from build123d import *

# Parameters (mm, degrees)
SKETCH_1_W      = 30
SKETCH_1_H      = 3
EXTRUDE_1_DEPTH = 3


with BuildPart() as part:
    # Эскиз1 → Бобышка-Вытянуть1 (new body)
    with BuildSketch(Plane.XY):
        Polygon((-25, 50), (-25, -50), (25, -50), (25, 50), (15, 50), (15, 47), (-15, 47), (-15, 50), align=None)
        with Locations((0, 48.5)):
            Rectangle(SKETCH_1_W, SKETCH_1_H)
        with Locations((0, 51.5)):
            Rectangle(SKETCH_1_W, SKETCH_1_H)
    extrude(amount=EXTRUDE_1_DEPTH)


solid = part.part
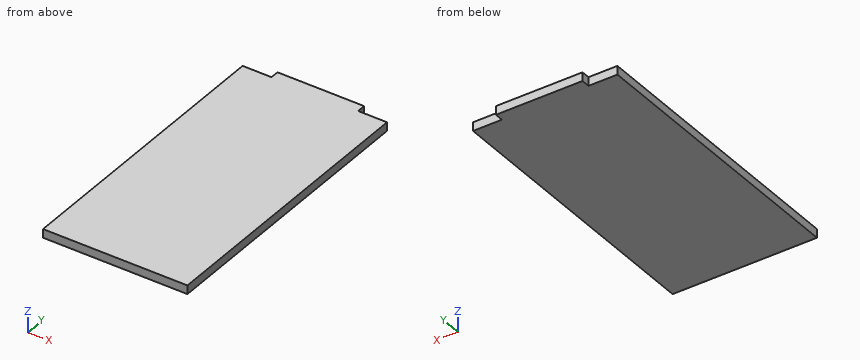
CAD build for the part. Positions are in the model's coordinates, mm. Coordinates: 2 decimals unless noted, no trailing zeros. Write each loop counter-clockwise with the first axis right and the second up, starting at its lowest first coordinate (ties: lowest second). Pieces come first, ordered by that corner, then holes. Notation, with made-up numbers: M 39.25,-25.75 L 76.25,-25.75 A30 cw 76.25,6.25 Z; hole C -26.5,89.5 d4. An arc over 180 degrees is marked long. Answer as a JSON object with one key per item and string values. Group by question number.
1) Pin check, flat tips, straight feed: pin 1 Ø0.9 at (y, z) = (52, 2) entering from -X; pin 2 Ø0.9 at (x, z) = (19, 2) entering from +Y. Stop position of each tip, or through.
2) Saw through at A-A (x = 16). Write the cut outline in (y, z), plus the area to 3 significant figures.
3) Wall check: line 1 (Y direction, x = 22, z = 2). Give the ranges that are in metal, low to high. Write a range as from..to.
Values follow:
{
 "1": {"pin 1": "stops at x = -15", "pin 2": "stops at y = 50"},
 "2": {"outline": "M -50,0 L 50,0 L 50,3 L -50,3 Z", "area": "300 mm2"},
 "3": {"line 1": "y = -50..50"}
}
